```python
from build123d import *

# Parameters (mm, degrees)
SKETCH1_W           = 127
SKETCH1_H           = 50.8
SKETCH1_R           = 2.5527
SKETCH1_R_2         = 3.429
BOSS_EXTRUDE1_DEPTH = 6.35
FILLET1_R           = 6.35


with BuildPart() as part:
    # Sketch1 → Boss-Extrude1 (new body)
    with BuildSketch(Plane(origin=(0, 0, 0), x_dir=(1, 0, 0), z_dir=(0, 1, 0))):
        with Locations((63.5, -25.4)):
            Rectangle(SKETCH1_W, SKETCH1_H)
        with Locations(Location((12.7, -12.7, 0), (0, 0, 270))):
            Circle(SKETCH1_R, mode=Mode.SUBTRACT)
        with Locations(Location((38.1, -12.7, 0), (0, 0, 270))):
            Circle(SKETCH1_R, mode=Mode.SUBTRACT)
        with Locations(Location((38.1, -38.1, 0), (0, 0, 270))):
            Circle(SKETCH1_R, mode=Mode.SUBTRACT)
        with Locations(Location((12.7, -38.1, 0), (0, 0, 270))):
            Circle(SKETCH1_R, mode=Mode.SUBTRACT)
        with Locations(Location((25.4, -25.4, 0), (0, 0, 270))):
            Circle(SKETCH1_R_2, mode=Mode.SUBTRACT)
        with Locations(Location((63.5, -25.4, 0), (0, 0, 270))):
            Circle(SKETCH1_R_2, mode=Mode.SUBTRACT)
        with Locations(Location((76.2, -25.4, 0), (0, 0, 270))):
            Circle(SKETCH1_R_2, mode=Mode.SUBTRACT)
        with Locations(Location((88.9, -25.4, 0), (0, 0, 270))):
            Circle(SKETCH1_R_2, mode=Mode.SUBTRACT)
        with Locations(Location((101.6, -25.4, 0), (0, 0, 270))):
            Circle(SKETCH1_R_2, mode=Mode.SUBTRACT)
        with Locations(Location((114.3, -25.4, 0), (0, 0, 270))):
            Circle(SKETCH1_R_2, mode=Mode.SUBTRACT)
    extrude(amount=BOSS_EXTRUDE1_DEPTH)

    # Fillet1
    fillet1_edges = [part.edges().sort_by_distance(p)[0] for p in [
        (0, 3.175, 0),
        (127, 3.175, 0),
        (127, 3.175, 50.8),
        (0, 3.175, 50.8),
    ]]
    fillet(fillet1_edges, radius=FILLET1_R)


solid = part.part
```
Model file for the job. Use its own axes, mm. Give positions to 0.01 mm unless a question says otherwise; leave off trailing zeros. Loops run counter-clockwise (first coordinate to the right, second up) from the corner with the lowest first, then second, coordinate; pieces in that order, holes last. Notation, with made-up numbers: (25.5, 12.5) -> (84.5, 12.5) arc R34 cw to (84.5, 45.5) -> close; hole circle Ø2 at (-6.75, 46.25). An arc over 180 degrees is marked (long way). Write each question's results on one line, items separated by ' | '.
(1) Flat gauge pin, fed straight in: pin 1 Ø11 at (x, z) = (76.2, 25.4) entering from -Y. Where does the tip first touch, or does it go through?
Geometry results:
pin 1: stops at y = 0
(2) Probe line 1 along X through (y, z) = (1.75, 12.7); line 2 along X through (y, z) = (4.75, 13); line 3 along Z through (x, y) = (103, 5.5). List the from-to ranges inside material, lowest first.
Geometry results:
line 1: x = 0 to 10.15, 15.25 to 35.55, 40.65 to 127 | line 2: x = 0 to 10.16, 15.24 to 35.56, 40.64 to 127 | line 3: z = 0 to 22.27, 28.53 to 50.8
(3) Cut at A-A on x = 12.7. List the corners of the cut face in (y, z).
Geometry results:
outline: (0, 0) -> (6.35, 0) -> (6.35, 10.15) -> (0, 10.15) -> close; (0, 15.25) -> (6.35, 15.25) -> (6.35, 35.55) -> (0, 35.55) -> close; (0, 40.65) -> (6.35, 40.65) -> (6.35, 50.8) -> (0, 50.8) -> close
(4) Cut at C-C on x = 88.9. List the corners of the cut face in (y, z).
Geometry results:
outline: (0, 0) -> (6.35, 0) -> (6.35, 21.97) -> (0, 21.97) -> close; (0, 28.83) -> (6.35, 28.83) -> (6.35, 50.8) -> (0, 50.8) -> close
(5) Cut at B-B on y = 4.5. Give the number of separate pieces and of enclosed holes in the cut face, and give its area (3 significant figures).
Geometry results:
separate pieces: 1 | enclosed holes: 10 | area: 6,110 mm²
(6) Cut at D-D on z = 39.5. List the corners of the cut face in (x, y).
Geometry results:
outline: (0, 0) -> (10.57, 0) -> (10.57, 6.35) -> (0, 6.35) -> close; (14.83, 0) -> (35.97, 0) -> (35.97, 6.35) -> (14.83, 6.35) -> close; (40.23, 0) -> (127, 0) -> (127, 6.35) -> (40.23, 6.35) -> close
(7) Pull direction Z, two halves, no side cores. Call faces 1 (the cylindrical face through (110.95, 3.13, 24.66)), 2 (the flat face through (127, 3, 26)), 3 (the flat face through (63, 3, 50.8)): released by +Z, released by -Z, zero draft, split by the parting line, or undercut.
Geometry results:
face 1: undercut | face 2: zero draft | face 3: released by +Z
